The listing builds one solid part. Answer for the finished solid, in the listing's coordinates (mm). A direction names the side the tool comes from. Round coordinates to 2 decimals unless told otherwise and drop trailing zeros. Write each loop counter-clockwise with the first axis right and the second up, starting at its lowest first coordinate (ties: lowest second). Pieces come first, ordered by that corner, then holes.
Autodesk Inventor part; units mm, degrees
ref_plane "YZ Plane" through (0, 0, 0) normal (1, 0, 0) x (0, 1, 0)
ref_plane "XZ Plane" through (0, 0, 0) normal (0, 1, 0) x (-1, 0, 0)
ref_plane "XY Plane" through (0, 0, 0) normal (0, 0, 1) x (1, 0, 0)
sketch "Sketch1" plane through (0, 0, 0) normal (0, 0, 1) x (1, 0, 0)
  circle A0 centre (0, 0) radius 6.9
  line L0 (0, 0) -> (0, 9.7668)
  circle A1 centre (0, 0) radius 4
  circle A2 centre (0, 4) radius 1.5
  circle A3 centre (-3.4641, -2) radius 1.5
  circle A4 centre (3.4641, -2) radius 1.5
  dimension "d1" = 8
  dimension "d0" = 13.8
  dimension "d2" = 3
  dimension "d5" = 360
extrude "Extrusion1" add sketch "Sketch1" along normal blind 4.53 contours A0 | A2 A1 A4 A3 | A3 A1 | A1 A3
sketch "Sketch2" plane through (0, 0, 4.53) normal (0, 0, 1) x (1, 0, 0)
  circle A0 centre (0, 0) radius 4.95
  dimension "d9" = 9.9
extrude "Extrusion2" add sketch "Sketch2" along normal blind 2.3
sketch "Sketch3" plane through (0, 0, 6.83) normal (0, 0, 1) x (1, 0, 0)
  circle A0 centre (0, 0) radius 3.05
  dimension "d12" = 6.1
extrude "Extrusion3" cut sketch "Sketch3" against normal blind 2.5
sketch "Sketch4" plane through (0, 0, 6.83) normal (0, 0, 1) x (1, 0, 0)
  arc A0 (1.2803, 4.7816) -> (-1.2803, 4.7816) centre (0, 4) ccw
  circle A1 centre (0, 4) radius 2.75
  circle A2 centre (-3.4641, -2) radius 2.75
  circle A3 centre (3.4641, -2) radius 2.75
  point P0 (0, 0)
  dimension "d15" = 5.5
  dimension "d18" = 360
extrude "Extrusion4" cut sketch "Sketch4" against normal blind 5.6 contours A1 | A3
chamfer "Chamfer1" distance 0.2 angle 45 2 edges at (2.6414, 1.525, 4.33) (-2.6414, -1.525, 4.33)
chamfer "Chamfer2" distance 0.2 angle 45 2 edges at (4.2868, 2.475, 6.83) (-4.2868, -2.475, 6.83)
chamfer "Chamfer3" distance 0.2 angle 45 4 edges at (-1.5, 4, 1.23) (0, 1.25, 4.33) (1.0825, -0.625, 4.33) (1.9641, -2, 1.23)
chamfer "Chamfer4" distance 0.2 angle 45 2 edges at (4.2868, 2.475, 4.53) (-4.2868, -2.475, 4.53)
properties part number "acc_motor_maghold"
1. Section C-C on z = 1.75 is taken. Determine the outline of the cut face in (x, y), plus the area to 3 significant figures.
Geometry says:
outline: circle Ø13.8 at (0, 0); hole circle Ø5.5 at (0, 4); hole circle Ø5.5 at (3.46, -2)
area: 102 mm2
2. Straight lines are drawn through the part: line 1 along Y through (x, z) = (1.5, 2.75); line 2 along Z through (x, y) = (0, 1.5); line 3 along X through (y, z) = (4, 3.1). For each, find the intervals that lie inside material, in ascending order.
Geometry says:
line 1: y = -6.73 to -3.92, -0.08 to 1.7, 6.3 to 6.73
line 2: z = 0 to 1.23
line 3: x = -5.62 to -2.75, 2.75 to 5.62
3. Given pin 1 (3 mm diameter, centred on x = 3, y = -1, fed in from +Z); pin 2 (1.5 mm diameter, centred on x = -5, y = -3, fed in from +Z); pin 3 (2.5 mm diameter, centred on x = 0, y = -1, fed in from +Z), each flat-ended and moving along its own axis, determine where each tip first touches the part or whether it passes through.
Geometry says:
pin 1: stops at z = 1.23
pin 2: stops at z = 4.6
pin 3: stops at z = 4.33
4. Section A-A on x = 0 is taken. Determine the outline of the cut face in (y, z).
Geometry says:
outline: (-6.9, 0) - (2.5, 0) - (2.5, 1.03) - (2.3, 1.23) - (1.25, 1.23) - (1.25, 4.13) - (1.05, 4.33) - (-2.85, 4.33) - (-3.05, 4.53) - (-3.05, 6.83) - (-4.75, 6.83) - (-4.95, 6.63) - (-4.95, 4.73) - (-5.15, 4.53) - (-6.9, 4.53) - close; (5.5, 0) - (6.9, 0) - (6.9, 4.53) - (6.75, 4.53) - (6.75, 1.23) - (5.7, 1.23) - (5.5, 1.03) - close
5. Section B-B on z = 5.75 is taken. Determine the outline of the cut face in (x, y).
Geometry says:
outline: (-2.75, 4.12) arc R4.95 ccw to (2.19, -4.44) arc R2.75 cw to (0.87, -2.92) arc R3.05 cw to (-2.09, 2.22) arc R2.75 cw to start; (2.09, 2.22) arc R3.05 cw to (2.97, 0.7) arc R2.75 cw to (4.94, 0.32) arc R4.95 ccw to (2.75, 4.12) arc R2.75 cw to start
6. A tool of negligible diameter and unlimited length cuts with its end or side. For faces 1 (the face through (-3, -2, 6.83)), 2 (the face through (3, -4, 1.23)), from which of +Z, -Z, +X, -X, +Y, -Y can it reach the whole face along a straight path? Write none if from no direction.
Geometry says:
face 1: +Z, +X, -X, +Y, -Y
face 2: +Z
7. For a pull along X with two mould halves and no side action, classify faces 3 (the face through (-3, -5, 4.53)), 4 (the face through (-0.9, -6.84, 2.23)), 5 (the face through (1.44, -0.14, 3.45)) as released by +X, released by -X, zero draft, split by the parting line, or undercut.
Geometry says:
face 3: zero draft
face 4: split by the parting line
face 5: undercut
